Verification items for the finished model (mm, model axes). A direction names the side the tool comes from. Give positions to 0.01 mm unless a question says otherwise; leave off trailing zeros. Loops run counter-clockwise (first coordinate to the right, second up) from the corner with the lowest first, then second, coordinate; pieces in that order, holes last. Notation, with made-up numbers: (51, 58) - (59, 58) arc R10 ccw to (59, 76) - close; hole circle Ø9 at (-2.75, 22). An arc over 180 degrees is marked (long way). Use one line per item in the form item = value.
```python
from build123d import *

# Parameters (mm, degrees)
F2_R     = 7.9375
F3_DEPTH = 25.4
F4_R     = 12.7
F4_R_2   = 7.9375
F5_DEPTH = 6.35


with BuildPart() as f1:
    # F0 (on Right) → F1 (revolve)
    with BuildSketch(Plane.YZ):
        Polygon((0, 17), (0, 0), (25.4, 0), (25.4, 3), (14.4, 3), (14.4, 14), (25.4, 14), (25.4, 17), align=None)
    revolve(axis=Axis((0, 0, 8.5), (0, 0, -1)))

    # F2 (on face) → F3 (cut)
    with BuildSketch(Plane.XY.offset(17)):
        Circle(F2_R)
    extrude(amount=-F3_DEPTH, mode=Mode.SUBTRACT)

    # F4 (on face) → F5 (join)
    with BuildSketch(Plane(origin=(0, 0, 0), x_dir=(1, 0, 0), z_dir=(0, 0, -1))):
        Circle(F4_R)
        Circle(F4_R_2, mode=Mode.SUBTRACT)
    extrude(amount=F5_DEPTH)


solid = f1.part
```
1. Section check C-C, the plane z = 10.75. Record the cut outline in (x, y) (1 decimal).
Result set:
outline = circle Ø28.8 at (0, 0); hole circle Ø15.9 at (0, 0)
2. Scan lines: probe 1 along Z at (x, y) = (0.5, 23.5); probe 2 along X at (y, z) = (0, 2); probe 3 along X at (y, z) = (0, 7). Record each from-to range of solid material in increasing order.
Result set:
probe_1 = 0 to 3, 14 to 17
probe_2 = -25.4 to -7.94, 7.94 to 25.4
probe_3 = -14.4 to -7.94, 7.94 to 14.4
3. Section check A-A, the plane y = 0. Record the cut outline in (x, z).
Result set:
outline = (-25.4, 0) - (-12.7, 0) - (-12.7, -6.35) - (-7.94, -6.35) - (-7.94, 17) - (-25.4, 17) - (-25.4, 14) - (-14.4, 14) - (-14.4, 3) - (-25.4, 3) - close; (7.94, -6.35) - (12.7, -6.35) - (12.7, 0) - (25.4, 0) - (25.4, 3) - (14.4, 3) - (14.4, 14) - (25.4, 14) - (25.4, 17) - (7.94, 17) - close
4. Tool access check on faces 4 (the flat face through (12, -5, 0)), 5 (the flat face through (6, -6, 17)), 6 (the cylindrical face through (4.325, 13.735, 8.577)). Record the directions out of +Z, -Z, +X, -X, +Y, -Y that give a thin tool (end or side, any length) a straight path to the whole face; none if there is none.
Result set:
face_4 = -Z
face_5 = +Z, +X, -X, +Y, -Y
face_6 = none
5. Depth check by flat-ended pin: pin 1 Ø8 at (y, z) = (10.5, 2.5) entering from +X; pin 2 Ø2 at (y, z) = (6.5, 12.5) entering from -X; pin 3 Ø8 at (x, z) = (4, -2) entering from -Y. Enter the tip coordinate at first touch or a pass-through.
Result set:
pin_1 = 24.55
pin_2 = -13.31
pin_3 = -25.39
6. Section check D-D, the plane x = 21.5. Record the cut outline in (y, z).
Result set:
outline = (-13.52, 0) - (13.52, 0) - (13.52, 3) - (-13.52, 3) - close; (-13.52, 14) - (13.52, 14) - (13.52, 17) - (-13.52, 17) - close
7. Draft check along Z on faces 1 (the flat face through (-11, 11, 3)), 2 (the flat face through (-0.2, 8.3, -6.35)), 3 (the cylindrical face through (-1.72, 7.75, 5.49)). Enter one of: released by +Z, released by -Z, zero draft, split by the parting line, or undercut.
Result set:
face_1 = undercut
face_2 = released by -Z
face_3 = zero draft
